Verification items for the finished model (mm, model axes). A direction names the side the tool comes from. Coordinates: 2 decimals unless noted, no trailing zeros. Loops run counter-clockwise (first coordinate to the right, second up) from the corner with the lowest first, then second, coordinate; pieces in that order, holes last.
Q1. Mould release check, pull along Z, two halves, no side actions. Record for faces 1 (the face through (-6.39, -34.88, 3.13)), 2 (the face through (3.175, -39, 0)), 3 (the face through (0.04, -47.19, 2.15)): +Z half, -Z half, draft (parallel to the pull), parting line (faces both ways), or undercut.
Q2. Go/stop test with flat-tipped pins: P1, Ø2, axis at x = 2.5, z = -5, coming from the -Y side; P2, Ø1, axis at x = 0.5, z = -1, coming from the +Y side; P3, Ø10, axis at x = -1.5, y = 18.5, coming from the +Z side. Record where each tip stops, or that it passes through.
Q3. Sectioned sample at C-C (y = -33.5). Enter the section's corners in (x, z) (3 decimals), then the cut area to 3 significant figures.
Q4. Sectioned sample at A-A (x = 0). Enter the section's corners in (y, z) (3 decimals).
Q5. Sectioned sample at B-B (z = 2). Enter the section's corners in (x, y) (3 decimals).
Q6. Material ranges on probe 1 along X at (y, z) = (25, 5.25) (3 decimals); probe 2 along Y at (x, z) = (-1, 1.75); probe 3 along Z at (x, y) = (-4.5, 26), recorded low to high.
Q7. Access from +Z, -Z, +X, -X, +Y, -Y to the whole of each face (thin tool, end or side, straight path). Record for faces 4 (the face through (-3.175, -39, 0)), 5 (the face through (0.07, -21.21, 3.13)), 6 (the face through (6.31, -34.88, 3.13)).
```python
from build123d import *

# Parameters (mm, degrees)
F1_DEPTH = 6.35
F3_DEPTH = 6.35
F5_D     = 6.35
F6_R     = 5.08
F7_R     = 5.08
F8_SIZE  = 6.34999
F9_R     = 5.08
F10_R    = 0.635


# Not quite as in the source:
# - a fillet or chamfer is up to 0.001 mm smaller than in the source, because OpenCascade refuses the exact size
# - a feature names something its author has since deleted; it is built from what else it names


with BuildPart() as f1:
    # F0 (on Top) → F1 (new body)
    with BuildSketch(Plane.XY):
        Polygon((9.525, 38.1), (-9.525, 38.1), (-9.525, -38.1), (-3.175, -38.1), (-3.175, -50.8), (3.175, -50.8), (3.175, -38.1), (9.525, -38.1), align=None)
        with BuildLine():
            ThreePointArc((3.175, -18.0363506079), (0, -21.2113506079), (-3.175, -18.0363506079))
            Line((-3.175, -18.0363506079), (-3.175, 31.75))
            ThreePointArc((-3.175, 31.75), (0, 34.925), (3.175, 31.75))
            Line((3.175, 31.75), (3.175, -18.0363506079))
        make_face(mode=Mode.SUBTRACT)
    extrude(amount=F1_DEPTH)

    # F2 (on face) → F3 (join)
    with BuildSketch(Plane(origin=(0, 0, 0), x_dir=(1, 0, 0), z_dir=(0, 0, -1))):
        Polygon((3.175, 38.1), (3.175, 50.8), (-3.175, 50.8), (-3.175, 38.1), (-3.175, 27.132358402), (3.175, 27.132358402), align=None)
    extrude(amount=F3_DEPTH)

    # F5 (through all)
    with Locations(Plane(origin=(-3.175, 0, 0), x_dir=(0, -1, 0), z_dir=(-1, 0, 0))):
        with Locations((44.8514223099, 0)):
            Hole(F5_D / 2)

    # F6
    f6_edges = [f1.edges().sort_by_distance(p)[0] for p in [
        (0, -50.8, -6.35),
    ]]
    fillet(f6_edges, radius=F6_R)

    # F7
    f7_edges = [f1.edges().sort_by_distance(p)[0] for p in [
        (-9.525, 38.1, 3.175),
        (9.525, 38.1, 3.175),
    ]]
    fillet(f7_edges, radius=F7_R)

    # F8 (size 6.35 in the source; OpenCascade refuses exactly that, so slightly less here)
    f8_edges = [f1.edges().sort_by_distance(p)[0] for p in [
        (6.35, -38.1, 0),
        (-6.35, -38.1, 0),
    ]]
    chamfer(f8_edges, length=F8_SIZE)

    # F9
    f9_edges = [f1.edges().sort_by_distance(p)[0] for p in [
        (0, -27.132358, -6.35),
    ]]
    fillet(f9_edges, radius=F9_R)

    # F10
    f10_edges = [f1.edges().sort_by_distance(p)[0] for p in [
        (-3.175, -50.8, 2.54),
        (3.175, -50.8, 2.54),
        (-9.525, 0.634995, 0),
        (9.525, -2.54, 6.35),
    ]]
    fillet(f10_edges, radius=F10_R)


solid = f1.part
```
Geometry check:
1. face 1: -Z half
1. face 2: draft
1. face 3: undercut
2. P1: stops at y = -50
2. P2: stops at y = -27.13
2. P3: stops at z = 6.35
3. outline: (-9.525, 1.75) - (-3.175, 1.75) - (-3.175, -5.715) arc R0.635 ccw to (-2.54, -6.35) - (2.54, -6.35) arc R0.635 ccw to (3.175, -5.715) - (3.175, 1.75) - (9.525, 1.75) - (9.525, 5.715) arc R0.635 ccw to (8.89, 6.35) - (-8.89, 6.35) arc R0.635 ccw to (-9.525, 5.715) - close
3. area: 139 mm2
4. outline: (-50.8, -1.27) arc R5.08 ccw to (-45.72, -6.35) - (-32.212, -6.35) arc R5.08 ccw to (-27.132, -1.27) - (-27.132, 0) - (-21.211, 0) - (-21.211, 6.35) - (-50.8, 6.35) - close; (34.925, 0) - (37.465, 0) arc R0.635 ccw to (38.1, 0.635) - (38.1, 5.715) arc R0.635 ccw to (37.465, 6.35) - (34.925, 6.35) - close; hole circle Ø6.35 at (-44.851, 0)
5. outline: (-9.525, -33.75) - (-3.175, -33.75) - (-3.175, -42.386) - (3.175, -42.386) - (3.175, -33.75) - (9.525, -33.75) - (9.525, 33.02) arc R5.08 ccw to (4.445, 38.1) - (-4.445, 38.1) arc R5.08 ccw to (-9.525, 33.02) - close; (-3.175, -50.165) arc R0.635 ccw to (-2.54, -50.8) - (2.54, -50.8) arc R0.635 ccw to (3.175, -50.165) - (3.175, -47.317) - (-3.175, -47.317) - close; hole (-3.175, -18.036) arc R3.175 ccw to (3.175, -18.036) - (3.175, 31.75) arc R3.175 ccw to (-3.175, 31.75) - close
6. probe 1: x = -9.525 to -3.175, 3.175 to 9.525
6. probe 2: y = -50.8 to -47.5, -42.2 to -21.05, 34.76 to 38.1
6. probe 3: z = 0 to 6.35
7. face 4: -Z, -X, -Y
7. face 5: +Z, -Z
7. face 6: -Z, +X, -Y
